```python
from build123d import *

# Parameters (mm, degrees)
F1_DEPTH  = 6.35
F3_DEPTH  = 3.175
F6_DEPTH  = 3.175
F8_DEPTH  = 3.175
F10_DEPTH = 3.048
F4_R      = 7.3778565178
F11_DEPTH = 3.175
F12_R     = 3.6859176852
F13_DEPTH = 6.351


# Not quite as in the source:
# - a feature names something its author has since deleted; it is built from what else it names


with BuildPart() as f1:
    # F0 (on Top) → F1 (new body)
    with BuildSketch(Plane.XY):
        with BuildLine():
            ThreePointArc((-36.3712396262, 11.3464940865), (-5.738718073, -37.6653304098), (38.1, 0))
            ThreePointArc((38.1, 0), (37.6653304098, 5.738718073), (36.3712396262, 11.3464940865))
            ThreePointArc((36.3712396262, 11.3464940865), (31.5544319278, 21.3524665018), (24.0569263159, 29.5444461148))
            ThreePointArc((24.0569263159, 29.5444461148), (0, 38.1), (-24.0569263159, 29.5444461148))
            ThreePointArc((-24.0569263159, 29.5444461148), (-31.5544319278, 21.3524665018), (-36.3712396262, 11.3464940865))
        make_face()
        with BuildLine():
            ThreePointArc((24.0569263159, 29.5444461148), (31.5544319278, 21.3524665018), (36.3712396262, 11.3464940865))
            ThreePointArc((36.3712396262, 11.3464940865), (49.3746579826, 26.088688726), (44.1774778249, 45.0468139009))
            Line((44.1774778249, 45.0468139009), (24.0569263159, 29.5444461148))
        make_face()
        with BuildLine():
            ThreePointArc((-44.1774778249, 45.0468139009), (-49.3746579826, 26.088688726), (-36.3712396262, 11.3464940865))
            ThreePointArc((-36.3712396262, 11.3464940865), (-31.5544319278, 21.3524665018), (-24.0569263159, 29.5444461148))
            Line((-24.0569263159, 29.5444461148), (-44.1774778249, 45.0468139009))
        make_face()
    extrude(amount=-F1_DEPTH)

    # F2 (on Top) → F3 (join)
    with BuildSketch(Plane.XY):
        with BuildLine():
            add(Edge.make_bspline(
                [(10.16, 0), (10.16, 6.7242064297), (-5.08, 3.3621032148), (-20.32, 0), (-5.08, -3.3621032148), (10.16, -6.7242064297), (10.16, 0)],
                knots=[0, 0, 0, 2.0943951024, 2.0943951024, 4.1887902048, 4.1887902048, 6.2831853072, 6.2831853072, 6.2831853072], degree=2, weights=[1, 0.5, 1, 0.5, 1, 0.5, 1]))
        make_face()
    extrude(amount=F3_DEPTH)

    # F5 (on face) → F6 (cut)
    with BuildSketch(Plane.XY):
        with BuildLine():
            Line((-30.9908390045, 27.2659789771), (-43.804358691, 38.5895557702))
            ThreePointArc((-43.804358691, 38.5895557702), (-44.8770730118, 27.4905174143), (-37.3975988477, 19.2202795297))
            ThreePointArc((-37.3975988477, 19.2202795297), (-34.4250124692, 23.4269092732), (-30.9908390045, 27.2659789771))
        make_face()
        with BuildLine():
            ThreePointArc((37.3975988477, 19.2202795297), (44.8770730118, 27.4905174143), (43.804358691, 38.5895557702))
            Line((43.804358691, 38.5895557702), (30.9908390045, 27.2659789771))
            ThreePointArc((30.9908390045, 27.2659789771), (34.4250124692, 23.4269092732), (37.3975988477, 19.2202795297))
        make_face()
    extrude(amount=-F6_DEPTH, mode=Mode.SUBTRACT)

    # F7 (on face) → F8 (cut)
    with BuildSketch(Plane.XY):
        with BuildLine():
            Line((12.7, -21.9528563652), (0, -21.9528563652))
            Line((0, -21.9528563652), (-12.7, -21.9528563652))
            ThreePointArc((-12.7, -21.9528563652), (-7.2401700339, -26.9432924529), (0, -28.4579321742))
            ThreePointArc((0, -28.4579321742), (7.2401700339, -26.9432924529), (12.7, -21.9528563652))
        make_face()
    extrude(amount=-F8_DEPTH, mode=Mode.SUBTRACT)

    # F9 (on face) → F10 (join)
    with BuildSketch(Plane.XY.offset(-3.175)):
        Polygon((-4.0704635903, -21.9528563652), (-8.815612644, -21.9528563652), (-6.5379412845, -25.3327768296), align=None)
        Polygon((4.0704635903, -21.9528563652), (6.5379412845, -25.3327768296), (8.815612644, -21.9528563652), align=None)
    extrude(amount=F10_DEPTH)

    # F4 (on face) → F11 (join)
    with BuildSketch(Plane.XY):
        with Locations((-14.8994419724, 13.2605032995)):
            Circle(F4_R)
        with Locations((14.8994419724, 13.2605032995)):
            Circle(F4_R)
    extrude(amount=F11_DEPTH)

    # F12 (on face) → F13 (cut, through all)
    with BuildSketch(Plane.XY):
        with Locations((41.7184382677, 24.286089465)):
            Circle(F12_R)
    extrude(amount=-F13_DEPTH, mode=Mode.SUBTRACT)


solid = f1.part
```
Model file for the job. Use its own axes, mm. A direction names the side the tool comes from. Round coordinates to 2 decimals unless told otherwise and drop trailing zeros. Order: outer loops, then holes, each group sorted by start corner. A loop starts at its lowest first (then second) coordinate and runs counter-clockwise, first axis right, second up. Notation, with made-up numbers: M -6,-3.75 L 6,-3.75 A19 ccw 6,31.25 Z; hole C 30,-15.5 d5. An arc over 180 degrees is marked long. Use CSV: the item, a comma, the result in double quotes.
Item 1: Saw through at B-B (y = -8). List the corners of the cut face in (x, z).
Worked answers:
outline,"M -37.25,-6.35 L 37.25,-6.35 L 37.25,0 L -37.25,0 Z"
Item 2: Pull direction X, two halves, no side cores. Call faces 4 (the face through (-15, 13, 3.175)), 5 (the face through (-44.927, 27.643, -1.565)), 6 (the face through (-49.437, 26.369, -3.131)): released by +X, released by -X, zero draft, split by the parting line, or undercut.
Worked answers:
face 4,"zero draft"
face 5,"undercut"
face 6,"released by -X"
Item 3: Which spindle directions (+Z, -Z, +X, -X, +Y, -Y) get a long thin tool onto all of the face, cutting with end or side? Do faces 1 (the face through (-1, 4, -6.35)), 2 (the face through (34.258, 37.404, -3.131)), 3 (the face through (34.38, 23.483, -1.565)). Say none if no direction does.
Worked answers:
face 1,"-Z, +X, -X, +Y, -Y"
face 2,"+Z, -Z, +Y"
face 3,"+Z"
Item 4: Saw through at C-C (x = -20.5). List the corners of the cut face in (y, z) (3 decimals), plus the area to 3 significant figures.
Worked answers:
outline,"M -32.115,-6.35 L 32.115,-6.35 L 32.115,0 L 18.063,0 L 18.063,3.175 L 8.458,3.175 L 8.458,0 L -32.115,0 Z"
area,"438 mm²"
Item 5: Pin check, flat tips, straight feed: pin 1 (2 mm diameter, centred on y = -22.5, z = 0, fed in from +X); pin 2 (4 mm diameter, centred on x = -0.5, y = 21, fed in from +Z); pin 3 (4 mm diameter, centred on x = -6, z = 0, fed in from +Y); pin 4 (6 mm diameter, centred on x = 41.72, y = 24.29, fed in from +Z). Stop position of each tip, or through.
Worked answers:
pin 1,"x = 31.45"
pin 2,"z = 0"
pin 3,"y = 37.89"
pin 4,"through"
Item 6: Saw through at D-D (y = -31). List the corners of the cut face in (x, z).
Worked answers:
outline,"M -22.15,-6.35 L 22.15,-6.35 L 22.15,0 L -22.15,0 Z"
Item 7: Probe probe 1 along Z at (x, y) = (27, 2.5); probe 2 along Z at (x, y) = (42, 33) (3 decimals); probe 3 along X at (y, z) = (-25, -1.25) (3 decimals). List the from-to ranges inside material, lowest first.
Worked answers:
probe 1,"-6.35 to 0"
probe 2,"-6.35 to -3.175"
probe 3,"-28.751 to -10.099, -6.762 to -6.295, 6.295 to 6.762, 10.099 to 28.751"
Item 8: Saw through at A-A (x = -33.5). List the corners of the cut face in (y, z) (3 decimals).
Worked answers:
outline,"M -18.148,-6.35 L 36.82,-6.35 L 36.82,0 L 29.483,0 L 29.483,-3.175 L 24.551,-3.175 L 24.551,0 L -18.148,0 Z"
